from build123d import *

# Parameters (mm, degrees)
F0_R     = 44.245933
F1_DEPTH = 39.624
F2_DEPTH = 13.208
F4_DEPTH = 11.43


with BuildPart() as f1:
    # F0 (on Top) → F1 (new body)
    with BuildSketch(Plane.XY):
        with BuildLine():
            ThreePointArc((52.940541, 78.661576), (-2.374099, 131.548857), (-52.72761, 73.918154))
            ThreePointArc((-52.72761, 73.918154), (0, 25.721035), (52.72761, 73.918154))
            ThreePointArc((52.72761, 73.918154), (52.887282, 76.287477), (52.940541, 78.661576))
        make_face()
        with Locations((0, 78.661576)):
            Circle(F0_R, mode=Mode.SUBTRACT)
    extrude(amount=F1_DEPTH)

    # F0 (on Top) → F2 (join)
    with BuildSketch(Plane.XY):
        with BuildLine():
            Line((-52.72761, 73.918154), (-52.72761, -78.661576))
            Line((-52.72761, -78.661576), (52.72761, -78.661576))
            Line((52.72761, -78.661576), (52.72761, 73.918154))
            ThreePointArc((52.72761, 73.918154), (0, 25.721035), (-52.72761, 73.918154))
        make_face()
    extrude(amount=F2_DEPTH)

    # F3 (on Right) → F4 (join, symmetric)
    with BuildSketch(Plane.YZ):
        Polygon((26.024748, 13.373829), (26.024748, 40.362455), (0, 13.373829), align=None)
    extrude(amount=F4_DEPTH, both=True)


solid = f1.part
The model under review builds one solid part; all positions refer to its coordinate system, in mm. A direction names the side the tool comes from. Give positions to 0.01 mm unless a question says otherwise; leave off trailing zeros. Order: outer loops, then holes, each group sorted by start corner. A loop starts at its lowest first (then second) coordinate and runs counter-clockwise, first axis right, second up. Notation, with made-up numbers: M 50.25,72 L 71.25,72 A18 ccw 71.25,92 Z; hole C 27.5,50 d6. An arc over 180 degrees is marked long. Answer in a Markdown table with one row per item. Add a question column.
1. Add section A-A on x = 0. State the section outline as (y, z) points, plus the area to 3 significant figures.
2. Add section B-B on y = 106. State the section outline as (x, z) points.
3. To check wall thickness, follow line 1 along Z through (x, y) = (-25, 1); line 2 along Y through (x, z) = (-36, 2.5); line 3 along X through (y, z) = (119.5, 24.5). State the ranges of each line that lie inside material, in increasing order.
4. Machinability: for faces 1 (the flat face through (-52.728, -1, 7)), 2 (the flat face through (-11.43, 19, 21)), 3 (the flat face through (52.728, -3, 7)), which of the approach directions +Z, -Z, +X, -X, +Y, -Y give a long, thin tool a straight path to every point of the face, cutting with its end or side? Answer none if there is none.
5. For pin 1 Ø2 at (x, y) = (-19, -52) entering from +Z; pin 2 Ø10.5 at (y, z) = (-39.5, 5.5) entering from -X; pin 3 Ø8 at (x, z) = (14.5, 33.5) entering from +Y; pin 4 Ø1 at (x, y) = (22.5, -36) entering from -Z, all flat-tipped, find the tip position at first contact; note any pin that passes through.
6. Mouldability with a two-part tool opening along Z and no side actions: class faces 4 (the flat face through (-1, 5, 0)), 5 (the flat face through (0, 13, 13.374)), 6 (the flat face through (43, 67, 39.624)), 7 (the flat face through (11.43, 19, 21)) as released by +Z, released by -Z, zero draft, split by the parting line, or undercut.
7. Add section C-C on z = 10.5. State the section outline as (x, y) points, plus the area to 3 significant figures.
8. Add section D-D on y = 32.5. State the section outline as (x, z) points.
The answers:
| question | item | result |
|---|---|---|
| 1 | outline | M -78.66,0 L 34.42,0 L 34.42,39.62 L 26.02,39.62 L 26.02,40.36 L 0,13.37 L 25.72,13.37 L 25.72,13.21 L -78.66,13.21 Z; M 122.91,0 L 131.6,0 L 131.6,39.62 L 122.91,39.62 Z |
| 1 | area | 2,410 mm2 |
| 2 | outline | M -45.34,0 L -34.79,0 L -34.79,39.62 L -45.34,39.62 Z; M 34.79,0 L 45.34,0 L 45.34,39.62 L 34.79,39.62 Z |
| 3 | line 1 | 0 to 13.21 |
| 3 | line 2 | -78.66 to 52.94, 104.39 to 117.48 |
| 3 | line 3 | -33.69 to -17.03, 17.03 to 33.69 |
| 4 | face 1 | +Z, -Z, -X, -Y |
| 4 | face 2 | +Z, -X, -Y |
| 4 | face 3 | +Z, -Z, +X, -Y |
| 5 | pin 1 | z = 13.21 |
| 5 | pin 2 | x = -52.73 |
| 5 | pin 3 | y = 130.55 |
| 5 | pin 4 | z = 0 |
| 6 | face 4 | released by -Z |
| 6 | face 5 | undercut |
| 6 | face 6 | released by +Z |
| 6 | face 7 | zero draft |
| 7 | outline | M -52.73,-78.66 L 52.73,-78.66 L 52.73,73.92 A52.94 ccw 52.94,78.66 A52.94 ccw long -52.73,73.92 Z; hole C 0,78.66 d88.49 |
| 7 | area | 14,800 mm2 |
| 8 | outline | M -52.73,0 L 52.73,0 L 52.73,13.21 L 25.92,13.21 L 25.92,39.62 L -25.92,39.62 L -25.92,13.21 L -52.73,13.21 Z |
